Build history of the part. All positions in model axes, mm. Face numbers are marked on the shaded views. A direction names the side the tool comes from. Give positions to 0.01 mm unless a question says otherwise; leave off trailing zeros. Write each loop counter-clockwise with the first axis right and the second up, starting at its lowest first coordinate (ties: lowest second). Pieces come first, ordered by that corner, then holes. Notation, with made-up numbers: (33, 38.25) -> (70, 38.25) arc R27 cw to (70, 75.25) -> close; hole circle Ø9 at (76, 79.5). An arc over 180 degrees is marked (long way). One line per question, with ' | ' between items. Start each with the question number.
(1) Pin check, flat tips, straight feed: P1, Ø0.9, axis at x = 20.5, z = 20, coming from the +Y side; P2, Ø0.8, axis at y = 25.5, z = 2, coming from the -X side; P3, Ø12, axis at x = 26, y = -2, coming from the +Z side; P4, Ø6, axis at x = 20, y = 13.5, coming from the +Z side. Stop position of each tip, or through.
(2) Band-saw the part on B-B, the plane z = 10. Give the cut face in (x, y).
(3) Pull direction Y, two halves, no side cores. Call the marked faces 1, 2, 3 and 4: released by +Y, released by -Y, zero draft, split by the parting line, or undercut.
(4) Tool access for the marked faces 5 and 6: list every direction of +Z, -Z, +X, -X, +Y, -Y with a clear straight run to the whole face (end or side of a thin tool).
(5) Drill centre lines: probe 1 along X at (y, z) = (19, 10.5); probe 2 along X at (y, z) = (7.5, 6); probe 3 along Y at (x, z) = (44, 2.4). Where is each one in solid material? Low to high. Write a range as from..to.
(6) Band-saw the part on C-C, the plane x = 31. Give the cut face in (y, z), and give its area (3 significant figures).
(7) Band-saw the part on A-A, the plane z = 5.15. Give the cut face in (x, y), and give its area (3 significant figures).
(8) Band-saw the part on D-D, the plane x = 43. Count the separate pieces of the cut face and the enclosed holes in it, and give its area (3 significant figures).
Autodesk Fusion 360 part; units mm, degrees
sketch "Esquisse1" plane through (0, 0, 0) normal (0, 0, 1) x (1, 0, 0)
  line L0 (0, 0) -> (59, 0)
  line L1 (59, 0) -> (59, 22)
  line L2 (59, 22) -> (0, 22)
  line L3 (0, 22) -> (0, 0)
  line L4 (0, 0) -> (0, 17) construction
  line L5 (0, 17) -> (0, 39) construction
  arc A0 (0, 17) -> (13.9642, 22) centre (0, 39) ccw
  dimension "d1" = 22
  dimension "d2" = 59
  dimension "d3" = 17
  dimension "d4" = 22
extrude "Extrusion1" add sketch "Esquisse1" along normal blind 2 contours L0 L1 L2 L3 A0
sketch "Esquisse2" plane through (0, 0, 2) normal (0, 0, 1) x (-1, 0, 0)
  line L0 (0, 0) -> (-59, 0)
  line L1 (-59, 0) -> (-59, -22)
  line L2 (-59, -22) -> (-13.9642, -22)
  arc A0 (0, -17) -> (-13.9642, -22) centre (0, -39) ccw
  line L3 (0, -17) -> (0, 0)
  arc A1 (-2, -15.0835) -> (-14.6629, -20) centre (0, -39) ccw
  line L4 (-57, -20) -> (-14.6629, -20)
  line L5 (-57, -2) -> (-57, -20)
  line L6 (-2, -2) -> (-57, -2)
  line L7 (-2, -15.0835) -> (-2, -2)
  dimension "d7" = -2
extrude "Extrusion2" add sketch "Esquisse2" along normal blind 19
sketch "Esquisse3" plane through (0, 0, 0) normal (-1, 0, 0) x (0, -1, 0)
  line L0 (-17, 0) -> (0, 0)
  line L1 (0, 0) -> (0, 21)
  line L2 (0, 21) -> (-17, 21)
  line L3 (-17, 21) -> (-17, 0)
  line L4 (-17, 7) -> (0, 7) construction
  circle A0 centre (-8.5, 7) radius 1.85 construction
  circle A1 centre (-8.4986, 5.15) radius 1.25
  circle A2 centre (-6.8986, 7.9263) radius 1.25
  circle A3 centre (-10.1029, 7.9237) radius 1.25
  dimension "d11" = 7
  dimension "d12" = 3.7
  dimension "d13" = 2.5
  dimension "d15" = 360
extrude "Extrusion3" cut sketch "Esquisse3" against normal blind 2 contours A1 | A2 | A3
sketch "Esquisse5" plane through (59, 0, 0) normal (1, 0, 0) x (0, 1, 0)
  line L0 (0, 0) -> (22, 0)
  line L1 (22, 0) -> (22, 21)
  line L2 (22, 21) -> (0, 21)
  line L3 (0, 21) -> (0, 0)
  circle A0 centre (11, 10) radius 3.25
  circle A1 centre (11, 10) radius 2
  dimension "d24" = 6.5
  dimension "d28" = 11
  dimension "d29" = 10
  dimension "d36" = 4
sketch "Esquisse6" plane through (0, 0, 2) normal (0, 0, 1) x (-1, 0, 0)
  line L0 (-2, -2) -> (-57, -2)
  line L1 (-57, -2) -> (-57, -20)
  line L2 (-57, -20) -> (-14.6629, -20)
  arc A0 (-2, -15.0835) -> (-14.6629, -20) centre (0, -39) ccw
  line L3 (-2, -15.0835) -> (-2, -2)
  line L4 (-57, -20) -> (-47, -20)
  line L5 (-47, -20) -> (-47, -2)
  line L6 (-47, -2) -> (-57, -2)
  line L7 (-57, -2) -> (-57, -20)
  dimension "d25" = 10
extrude "Extrusion5" add sketch "Esquisse6" along normal blind 12 contours L0 L1 L2 L4 L5 L6 L7
extrude "Extrusion6" cut sketch "Esquisse5" against normal blind 19 contours A0 | A1
sketch "Esquisse7" plane through (0, 0, 14) normal (0, 0, 1) x (-1, 0, 0)
  line L0 (-57, -2) -> (-57, -20)
  line L1 (-57, -20) -> (-47, -20)
  line L2 (-47, -20) -> (-47, -2)
  line L3 (-57, -20) -> (-57, -2)
  line L4 (-57, -20) -> (-51, -20)
  line L5 (-51, -20) -> (-51, -2)
  line L6 (-51, -2) -> (-57, -2)
  line L7 (-57, -2) -> (-57, -20)
  line L8 (-47, -2) -> (-57, -2)
  dimension "d35" = 6
extrude "Extrusion7" cut sketch "Esquisse7" against normal blind 10 contours L0 L1 L3 L4 L5 L6 L7 L8
extrude "Extrusion8" cut sketch "Esquisse5" against normal blind 13 contours A1
sketch "Esquisse8" plane through (51, 0, 0) normal (1, 0, 0) x (0, 1, 0)
  line L0 (20, 14) -> (2, 14)
  line L1 (2, 14) -> (2, 4)
  line L2 (2, 4) -> (20, 4)
  line L3 (20, 4) -> (20, 14)
  circle A0 centre (11, 10) radius 3.25
sketch "Esquisse9" plane through (0, 0, 0) normal (0, 0, -1) x (1, 0, 0)
  line L0 (59, 0) -> (0, 0)
  line L1 (0, 0) -> (0, -17)
  arc A0 (13.9642, -22) -> (0, -17) centre (0, -39) ccw
  line L2 (13.9642, -22) -> (59, -22)
  line L3 (59, -22) -> (59, 0)
  line L4 (40, 0) -> (48, 0)
  line L5 (48, 0) -> (48, 8)
  line L6 (48, 8) -> (40, 8)
  line L7 (40, 8) -> (40, 0)
  line L8 (44, 0) -> (44, 8) construction
  line L9 (59, -11) -> (19, -11) construction
  line L10 (48, -22) -> (48, -30)
  line L11 (48, -30) -> (40, -30)
  line L12 (40, -30) -> (40, -22)
  line L13 (40, -22) -> (48, -22)
  circle A1 centre (44, 4) radius 1.7
  circle A2 centre (44, -26) radius 1.7
  dimension "d39" = 8
  dimension "d40" = 8
  dimension "d41" = 15
  dimension "d44" = 3.4
extrude "Extrusion9" add sketch "Esquisse9" against normal blind 3 contours L0 L4 L5 L6 L7 | L2 L10 L11 L12 L13
fillet "Congé1" radius 4 4 edges at (48, -8, 1.5) (40, -8, 1.5) (48, 30, 1.5) (40, 30, 1.5)
fillet "Congé2" radius 3 4 edges at (48, 0, 1.5) (48, 22, 1.5) (40, 22, 1.5) (40, 0, 1.5)
sketch "Esquisse10" plane through (0, 0, 21) normal (0, 0, 1) x (-1, 0, 0)
  line L0 (-2, -2) -> (-2, -15.0835)
  arc A0 (-2, -15.0835) -> (-14.6629, -20) centre (0, -39) ccw
  line L1 (-14.6629, -20) -> (-57, -20)
  line L2 (-57, -20) -> (-57, -2)
  line L3 (-57, -2) -> (-2, -2)
  line L4 (0, -17) -> (0, 0)
  line L5 (0, 0) -> (-59, 0)
  line L6 (-59, 0) -> (-59, -22)
  line L7 (-59, -22) -> (-13.9642, -22)
  arc A1 (0, -17) -> (-13.9642, -22) centre (0, -39) ccw
  line L8 (-57.8, -1.2) -> (-1.2, -1.2)
  line L9 (-1.2, -1.2) -> (-1.2, -15.8311)
  arc A2 (-1.2, -15.8311) -> (-14.3875, -20.8) centre (0, -39) ccw
  line L10 (-14.3875, -20.8) -> (-57.8, -20.8)
  line L11 (-57.8, -20.8) -> (-57.8, -1.2)
  dimension "d49" = -0.8
extrude "Extrusion10" cut sketch "Esquisse10" against normal blind 2 contours L8 L9 A2 L10 L11
chamfer "Chanfrein1" distance 0.2 angle 45 5 edges at (8.1802, 17.29, 21) (36.0937, 20.8, 21) (57.8, 11, 21) (29.5, 1.2, 21) (1.2, 8.5155, 21)
fillet "Congé3" radius 1.5 3 edges at (0, 0, 10.5) (59, 0, 10.5) (59, 22, 10.5)
fillet "Congé4" radius 1 2 edges at (0, 17, 10.5) (13.9642, 22, 10.5)
chamfer "Chanfrein2" distance 0.5 angle 45 2 edges at (51, 11, 14) (47, 11, 14)
hole "Perçage1" at (44, -4, 3) direction (0, 0, -1) diameter 6 depth 1.5 tip angle 180
hole "Perçage2" at (44, 26, 3) direction (0, 0, -1) diameter 6 depth 1.5 tip angle 180
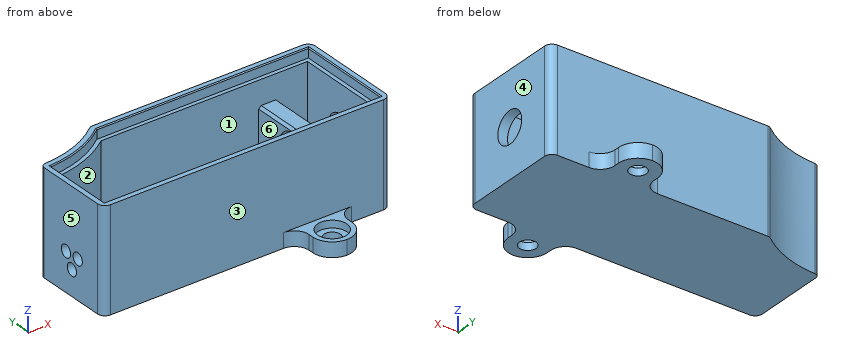
Results:
1) P1: stops at y = 22 | P2: stops at x = 40 | P3: stops at z = 21 | P4: stops at z = 2
2) outline: (0, 1.5) arc R1.5 ccw to (1.5, 0) -> (57.5, 0) arc R1.5 ccw to (59, 1.5) -> (59, 7.75) -> (57, 7.75) -> (57, 2) -> (51, 2) -> (51, 7.75) -> (47, 7.75) -> (47, 2) -> (2, 2) -> (2, 15.08) arc R24 ccw to (14.66, 20) -> (47, 20) -> (47, 14.25) -> (51, 14.25) -> (51, 20) -> (57, 20) -> (57, 14.25) -> (59, 14.25) -> (59, 20.5) arc R1.5 ccw to (57.5, 22) -> (14.32, 22) arc R1 ccw to (13.7, 21.78) arc R22 cw to (0.96, 17.02) arc R1 ccw to (0, 16.02) -> close
3) face 1: undercut | face 2: undercut | face 3: released by -Y | face 4: zero draft
4) face 5: +Z, -Z, -X, +Y, -Y | face 6: +Z
5) probe 1: x = 9.17..13.27, 47..51, 57..59 | probe 2: x = 0..2, 47..51, 57..59 | probe 3: y = -8..-7, -1..2, 20..23, 29..30
6) outline: (0, 0) -> (22, 0) -> (22, 21) -> (21, 21) -> (20.8, 20.8) -> (20.8, 19) -> (20, 19) -> (20, 2) -> (2, 2) -> (2, 19) -> (1.2, 19) -> (1.2, 20.8) -> (1, 21) -> (0, 21) -> close | area: 117 mm²
7) outline: (0, 1.5) arc R1.5 ccw to (1.5, 0) -> (57.5, 0) arc R1.5 ccw to (59, 1.5) -> (59, 20.5) arc R1.5 ccw to (57.5, 22) -> (14.32, 22) arc R1 ccw to (13.7, 21.78) arc R22 cw to (0.96, 17.02) arc R1 ccw to (0, 16.02) -> (0, 9.75) -> (2, 9.75) -> (2, 15.08) arc R24 ccw to (14.66, 20) -> (47, 20) -> (47, 2) -> (2, 2) -> (2, 7.25) -> (0, 7.25) -> close; hole (51, 2) -> (57, 2) -> (57, 20) -> (51, 20) -> close | area: 366 mm²
8) separate pieces: 3 | enclosed holes: 0 | area: 139 mm²
